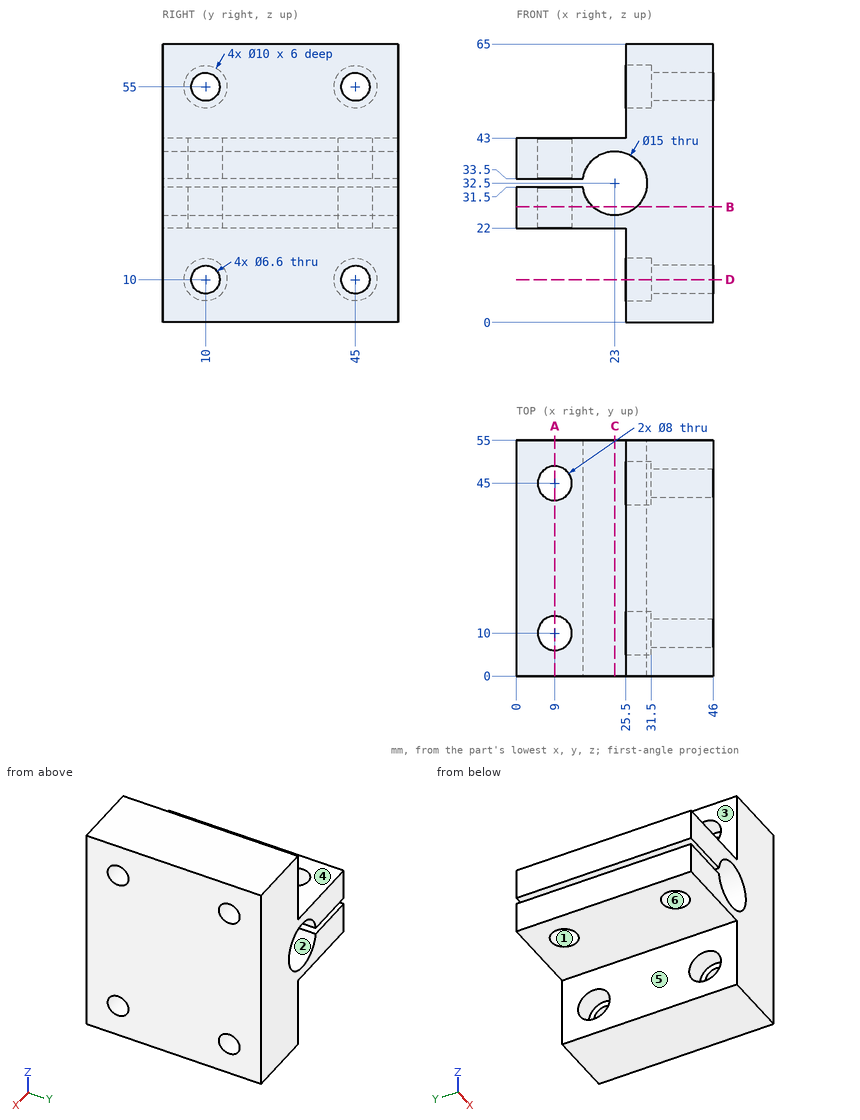
Verification items for this drawing (mm, ordinates from the low corner). A direction names the side the tool comes from. Round coordinates to 2 decimals unless told otherwise and drop trailing zeros. Order: outer loops, then holes, each group sorted by start corner. A loop starts at its lowest first (then second) coordinate and runs counter-clockwise, first axis right, second up. Notation, with made-up numbers: (32.25, -36) - (40.25, -36) arc R10 cw to (40.25, -30) - close; hole circle Ø10 at (24.25, 76.25). An arc over 180 degrees is marked (long way). Answer as CSV lines item,"result". Start each with the question number.
1) Tool access check on the marked faces 5 and 6. Record the directions out of +Z, -Z, +X, -X, +Y, -Y that give a thin tool (end or side, any length) a straight path to the whole face; none if there is none.
2) Section check D-D (z = 10). Record the cut outline in (x, y).
3) Section check C-C (x = 23). Record the cut outline in (y, z).
4) Section check A-A (x = 9). Record the cut outline in (y, z), then the cut area to 3 significant figures.
5) Section check B-B (z = 27). Record the cut outline in (x, y), then the cut area to 3 significant figures.
6) Draft check along X on the marked faces 1, 2, 3 and 4. Enter one of: +X half, -X half, draft (parallel to the pull), parting line (faces both ways), or undercut.
7) Depth check by flat-ended pin: pin 1 (5 mm diameter, centred on y = 8.5, z = 54.5, fed in from -X); pin 2 (10.5 mm diameter, centred on x = 9, y = 45, fed in from +Z); pin 3 (7.5 mm diameter, centred on x = 11.5, y = 40.5, fed in from -Z). Enter the tip coordinate at first touch or a pass-through.
8) Scan lines: probe 1 along Z at (x, y) = (41.5, 45); probe 2 along Z at (x, y) = (5, 5.5); probe 3 along X at (y, z) = (7, 34). Record each from-to range of solid material in increasing order.
Determined:
1,face 5,"-Z, -X, +Y, -Y"
1,face 6,"+Z, -Z"
2,outline,"(25.5, 0) - (46, 0) - (46, 6.7) - (31.5, 6.7) - (31.5, 5) - (25.5, 5) - close; (25.5, 15) - (31.5, 15) - (31.5, 13.3) - (46, 13.3) - (46, 41.7) - (31.5, 41.7) - (31.5, 40) - (25.5, 40) - close; (25.5, 50) - (31.5, 50) - (31.5, 48.3) - (46, 48.3) - (46, 55) - (25.5, 55) - close"
3,outline,"(0, 22) - (55, 22) - (55, 25) - (0, 25) - close; (0, 40) - (55, 40) - (55, 43) - (0, 43) - close"
4,outline,"(0, 22) - (6, 22) - (6, 31.5) - (0, 31.5) - close; (0, 33.5) - (6, 33.5) - (6, 43) - (0, 43) - close; (14, 22) - (41, 22) - (41, 31.5) - (14, 31.5) - close; (14, 33.5) - (41, 33.5) - (41, 43) - (14, 43) - close; (49, 22) - (55, 22) - (55, 31.5) - (49, 31.5) - close; (49, 33.5) - (55, 33.5) - (55, 43) - (49, 43) - close"
4,area,"741 mm^2"
5,outline,"(0, 0) - (17.9, 0) - (17.9, 55) - (0, 55) - close; (28.1, 0) - (46, 0) - (46, 55) - (28.1, 55) - close; hole circle Ø8 at (9, 10); hole circle Ø8 at (9, 45)"
5,area,"1,870 mm^2"
6,face 1,"undercut"
6,face 2,"undercut"
6,face 3,"-X half"
6,face 4,"draft"
7,pin 1,"x = 31.5"
7,pin 2,"z = 43"
7,pin 3,"z = 22"
8,probe 1,"0 to 6.7, 13.3 to 51.7, 58.3 to 65"
8,probe 2,"22 to 31.5, 33.5 to 43"
8,probe 3,"0 to 6.35, 11.65 to 15.65, 30.35 to 46"
